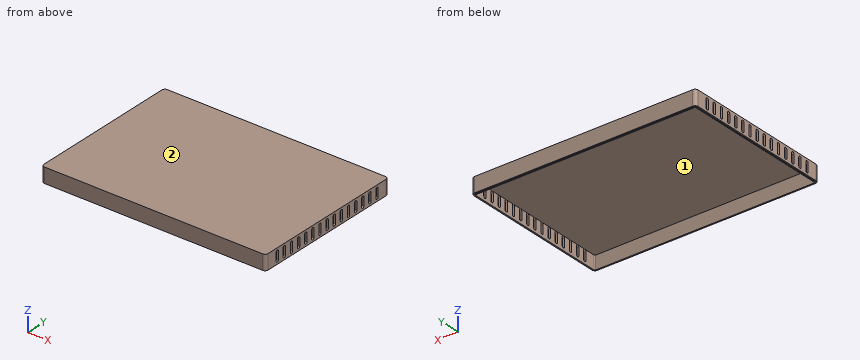
from build123d import *

# Parameters (mm, degrees)
SKETCH_1_W          = 225
SKETCH_1_H          = 155
EXTRUDE_1_DEPTH     = 15
FILLET_1_R          = 3
SHELL_1_T           = -2
EXTRUDE_2_DEPTH     = 0.5
CUT_EXTRUDE_1_DEPTH = 3


with BuildPart() as part:
    # 草图1 → 凸台-拉伸1 (new body)
    with BuildSketch(Plane.XY):
        with Locations((112.5, -77.5)):
            Rectangle(SKETCH_1_W, SKETCH_1_H)
    extrude(amount=EXTRUDE_1_DEPTH)

    # 圆角1
    fillet_1_edges = [part.edges().sort_by_distance(p)[0] for p in [
        (0, 0, 7.5),
        (225, 0, 7.5),
        (225, -155, 7.5),
        (0, -155, 7.5),
    ]]
    fillet(fillet_1_edges, radius=FILLET_1_R)

    # 抽壳1
    shell_1_openings = [part.faces().sort_by_distance(p)[0] for p in [
        (112.5, -77.5, 0),
    ]]
    offset(amount=SHELL_1_T, openings=shell_1_openings, kind=Kind.INTERSECTION)

    # 草图4 → 凸台-拉伸2 (add)
    with BuildSketch(Plane(origin=(0, 0, 0), x_dir=(-1, 0, 0), z_dir=(0, 0, -1))):
        with BuildLine():
            Line((-223.8, -3), (-223.8, -152))
            ThreePointArc((-223.8, -152), (-223.272792206, -153.272792206), (-222, -153.8))
            Line((-222, -153.8), (-3, -153.8))
            ThreePointArc((-3, -153.8), (-1.727207794, -153.272792206), (-1.2, -152))
            Line((-1.2, -152), (-1.2, -3))
            ThreePointArc((-1.2, -3), (-1.727207794, -1.727207794), (-3, -1.2))
            Line((-3, -1.2), (-222, -1.2))
            ThreePointArc((-222, -1.2), (-223.272792206, -1.727207794), (-223.8, -3))
        make_face()
        with BuildLine():
            Line((-223, -3), (-223, -152))
            ThreePointArc((-223, -152), (-222.707106781, -152.707106781), (-222, -153))
            Line((-222, -153), (-3, -153))
            ThreePointArc((-3, -153), (-2.292893219, -152.707106781), (-2, -152))
            Line((-2, -152), (-2, -3))
            ThreePointArc((-2, -3), (-2.292893219, -2.292893219), (-3, -2))
            Line((-3, -2), (-222, -2))
            ThreePointArc((-222, -2), (-222.707106781, -2.292893219), (-223, -3))
        make_face(mode=Mode.SUBTRACT)
    extrude(amount=EXTRUDE_2_DEPTH)

    # 草图5 → 切除-拉伸1 (cut)
    with BuildSketch(Plane.ZY):
        with BuildLine():
            Line((3.5, -13), (11.5, -13))
            ThreePointArc((11.5, -13), (13, -14.5), (11.5, -16))
            Line((11.5, -16), (3.5, -16))
            ThreePointArc((3.5, -16), (2, -14.5), (3.5, -13))
        make_face()
        with BuildLine():
            Line((3.5, -22), (11.5, -22))
            ThreePointArc((11.5, -22), (13, -23.5), (11.5, -25))
            Line((11.5, -25), (3.5, -25))
            ThreePointArc((3.5, -25), (2, -23.5), (3.5, -22))
        make_face()
        with BuildLine():
            Line((3.5, -31), (11.5, -31))
            ThreePointArc((11.5, -31), (13, -32.5), (11.5, -34))
            Line((11.5, -34), (3.5, -34))
            ThreePointArc((3.5, -34), (2, -32.5), (3.5, -31))
        make_face()
        with BuildLine():
            Line((3.5, -40), (11.5, -40))
            ThreePointArc((11.5, -40), (13, -41.5), (11.5, -43))
            Line((11.5, -43), (3.5, -43))
            ThreePointArc((3.5, -43), (2, -41.5), (3.5, -40))
        make_face()
        with BuildLine():
            Line((3.5, -49), (11.5, -49))
            ThreePointArc((11.5, -49), (13, -50.5), (11.5, -52))
            Line((11.5, -52), (3.5, -52))
            ThreePointArc((3.5, -52), (2, -50.5), (3.5, -49))
        make_face()
        with BuildLine():
            Line((3.5, -58), (11.5, -58))
            ThreePointArc((11.5, -58), (13, -59.5), (11.5, -61))
            Line((11.5, -61), (3.5, -61))
            ThreePointArc((3.5, -61), (2, -59.5), (3.5, -58))
        make_face()
        with BuildLine():
            Line((3.5, -67), (11.5, -67))
            ThreePointArc((11.5, -67), (13, -68.5), (11.5, -70))
            Line((11.5, -70), (3.5, -70))
            ThreePointArc((3.5, -70), (2, -68.5), (3.5, -67))
        make_face()
        with BuildLine():
            Line((3.5, -76), (11.5, -76))
            ThreePointArc((11.5, -76), (13, -77.5), (11.5, -79))
            Line((11.5, -79), (3.5, -79))
            ThreePointArc((3.5, -79), (2, -77.5), (3.5, -76))
        make_face()
        with BuildLine():
            Line((3.5, -85), (11.5, -85))
            ThreePointArc((11.5, -85), (13, -86.5), (11.5, -88))
            Line((11.5, -88), (3.5, -88))
            ThreePointArc((3.5, -88), (2, -86.5), (3.5, -85))
        make_face()
        with BuildLine():
            Line((3.5, -94), (11.5, -94))
            ThreePointArc((11.5, -94), (13, -95.5), (11.5, -97))
            Line((11.5, -97), (3.5, -97))
            ThreePointArc((3.5, -97), (2, -95.5), (3.5, -94))
        make_face()
        with BuildLine():
            Line((3.5, -103), (11.5, -103))
            ThreePointArc((11.5, -103), (13, -104.5), (11.5, -106))
            Line((11.5, -106), (3.5, -106))
            ThreePointArc((3.5, -106), (2, -104.5), (3.5, -103))
        make_face()
        with BuildLine():
            Line((3.5, -112), (11.5, -112))
            ThreePointArc((11.5, -112), (13, -113.5), (11.5, -115))
            Line((11.5, -115), (3.5, -115))
            ThreePointArc((3.5, -115), (2, -113.5), (3.5, -112))
        make_face()
        with BuildLine():
            Line((3.5, -121), (11.5, -121))
            ThreePointArc((11.5, -121), (13, -122.5), (11.5, -124))
            Line((11.5, -124), (3.5, -124))
            ThreePointArc((3.5, -124), (2, -122.5), (3.5, -121))
        make_face()
        with BuildLine():
            Line((3.5, -130), (11.5, -130))
            ThreePointArc((11.5, -130), (13, -131.5), (11.5, -133))
            Line((11.5, -133), (3.5, -133))
            ThreePointArc((3.5, -133), (2, -131.5), (3.5, -130))
        make_face()
        with BuildLine():
            Line((3.5, -139), (11.5, -139))
            ThreePointArc((11.5, -139), (13, -140.5), (11.5, -142))
            Line((11.5, -142), (3.5, -142))
            ThreePointArc((3.5, -142), (2, -140.5), (3.5, -139))
        make_face()
    cut_extrude_1 = extrude(amount=-CUT_EXTRUDE_1_DEPTH, mode=Mode.SUBTRACT)

    # 镜向1: 切除-拉伸1 across plane
    add(cut_extrude_1.mirror(Plane(origin=(112.5, 0, 0), x_dir=(0, 0, 1), z_dir=(1, 0, 0))), mode=Mode.SUBTRACT)


solid = part.part
Here's how the part is built. I have some questions about the finished solid (model axes, mm). Face numbers are marked on the shaded views. A direction names the side the tool comes from. Give positions to 0.01 mm unless a question says otherwise; leave off trailing zeros. Loops run counter-clockwise (first coordinate to the right, second up) from the corner with the lowest first, then second, coordinate; pieces in that order, holes last. Notation, with made-up numbers: (62.25, 70) -> (66.25, 70) arc R25 cw to (66.25, 96) -> close; hole circle Ø9 at (64, -15). An arc over 180 degrees is marked (long way). One line per item, written item: value.
Q1. Suppose I cut it at A-A on x = 159.5. Please give me the cut outline in (y, z).
Answers follow:
outline: (-155, 0) -> (-153.8, 0) -> (-153.8, -0.5) -> (-153, -0.5) -> (-153, 13) -> (-2, 13) -> (-2, -0.5) -> (-1.2, -0.5) -> (-1.2, 0) -> (0, 0) -> (0, 15) -> (-155, 15) -> close
Q2. If I drill on line 1 along X through (y, z) = (-97.5, 10); line 2 along Y through (x, z) = (196.5, 3.75); line 3 along Z through (x, y) = (192, -144), over which ranges is the centre line in solid material (lowest first)?
Answers follow:
line 1: 0 to 2, 223 to 225
line 2: -155 to -153, -2 to 0
line 3: 13 to 15
Q3. I'm going to push flat-ended pins straight in: pin 1 Ø2 at (x, z) = (224, 6.5) entering from -Y; pin 2 Ø0.6 at (x, z) = (224, 8.5) entering from +Y; pin 3 Ø2 at (x, z) = (224, 6.5) entering from +Y. Where does each tip first touch, or does it pass through?
Answers follow:
pin 1: y = -154.83
pin 2: y = -0.53
pin 3: y = -0.17
Q4. On a 3-axis mill with a long thin cutter (end or side, diameter ignored), from which of +Z, -Z, +X, -X, +Y, -Y can I reach the whole of each face in a straight line? I mean the marked faces 1 and 2. Say none if no direction works.
Answers follow:
face 1: -Z
face 2: +Z, +X, -X, +Y, -Y
